Geometry: final body of the model. Coordinates: model frame, mm. Give positions to 0.01 mm unless a question says otherwise; leave off trailing zeros. Write each loop counter-clockwise with the first axis right and the second up, starting at its lowest first coordinate (ties: lowest second). Pieces come first, ordered by that corner, then holes. Notation, with made-up numbers: (24, 27) -> (50, 27) arc R29 ccw to (50, 54) -> close; hole circle Ø10 at (-1, 36). An arc over 180 degrees is marked (long way). Answer as a JSON object with one key per item and string values. Group by question number.
(1) Material intervals for probe 1 along X at (y, z) = (0.3, -2.5); probe 2 along Z at (x, y) = (2, 0.45); probe 3 along Y at (x, z) = (7.75, -205.5), sorted ascending.
(2) Contact query for a flat-ended pin moving along its axis: pin 1 Ø1.4 at (x, z) = (2, -2.5) entering from -Y. Output: stop coordinate, or through.
(3) Section query A-A on z = -196. Output: boundary loops of the cut face in (x, y).
Autodesk Inventor part; units mm, degrees
ref_plane "YZ Plane" through (0, 0, 0) normal (1, 0, 0) x (0, 1, 0)
ref_plane "XZ Plane" through (0, 0, 0) normal (0, 1, 0) x (-1, 0, 0)
ref_plane "XY Plane" through (0, 0, 0) normal (0, 0, 1) x (1, 0, 0)
sketch "草图1" plane through (0, 0, 0) normal (0, 1, 0) x (-1, 0, 0)
  line L0 (0, 0) -> (-10, 0)
  line L1 (-10, 0) -> (-10, -400)
  line L2 (-10, -400) -> (0, -400)
  line L3 (0, -400) -> (0, 0)
  dimension "d0" = 10
  dimension "d1" = 400
extrude "拉伸1" add sketch "草图1" along normal blind 1
sketch "草图2" plane through (0, 1, 0) normal (0, 1, 0) x (1, 0, 0)
  circle A0 centre (2, 2.5) radius 1.5
  circle A1 centre (8, 2.5) radius 1.5
  line L0 (0, 400) -> (0, 0)
  line L1 (10, 0) -> (10, 400)
  line L2 (0, 0) -> (10, 0)
  dimension "d4" = 3
  dimension "d5" = 3
  dimension "d6" = 2
  dimension "d7" = 2
  dimension "d8" = 2.5
  dimension "d9" = 2.5
sketch "草图3" plane through (0, 1, 0) normal (0, 1, 0) x (1, 0, 0)
  point P0 (0, 0)
extrude "拉伸2" add sketch "草图2" along normal blind 0.1
sketch "草图4" plane through (2, 1.1, -2.5) normal (0, 1, 0) x (1, 0, 0)
  circle A0 centre (0, 0) radius 1.5
  circle A1 centre (0, 0) radius 0.75
  circle A2 centre (6, 0) radius 1.5
  circle A3 centre (6, 0) radius 0.75
  point P0 (-2, -2.5)
  dimension "d12" = 1.5
  dimension "d13" = 1.5
extrude "拉伸3" cut sketch "草图4" against normal blind 3.85 contours A1 | A3
sketch "草图5" plane through (0, 1, 0) normal (0, 1, 0) x (1, 0, 0)
  line L0 (3.0005, 45) -> (4.4505, 45)
  line L1 (4.4505, 45) -> (4.4505, 395)
  line L2 (4.4505, 395) -> (3.0005, 395)
  line L3 (3.0005, 395) -> (3.0005, 45)
  line L4 (5.5405, 45) -> (6.9905, 45)
  line L5 (6.9905, 45) -> (6.9905, 395)
  line L6 (6.9905, 395) -> (5.5405, 395)
  line L7 (5.5405, 395) -> (5.5405, 45)
  line L8 (0, 0) -> (10, 0)
  line L9 (10, 400) -> (0, 400)
  line L10 (0, 400) -> (0, 0)
  dimension "d16" = 1.45
  dimension "d17" = 350
  dimension "d18" = 1.45
  dimension "d19" = 350
  dimension "d20" = 45
  dimension "d21" = 5
  dimension "d22" = 1.09
  dimension "d23" = 3.0005
extrude "拉伸4" add sketch "草图5" along normal blind 0.1
equation "\"折弯半径\" = 厚度"
equation "\"折弯释压宽度\" = 厚度"
equation "\"折弯释压深度\" = 0.5 * 厚度"
equation "\"拐角释压尺寸\" = 4 * 厚度"
equation "\"最小余量\" = 2 * 厚度"
equation "\"过渡半径\" = 折弯半径"
equation "\"Jacobi半径尺寸\" = 折弯半径"
equation "\"间隙大小\" = 厚度"
properties part number "Dosyn Rail"
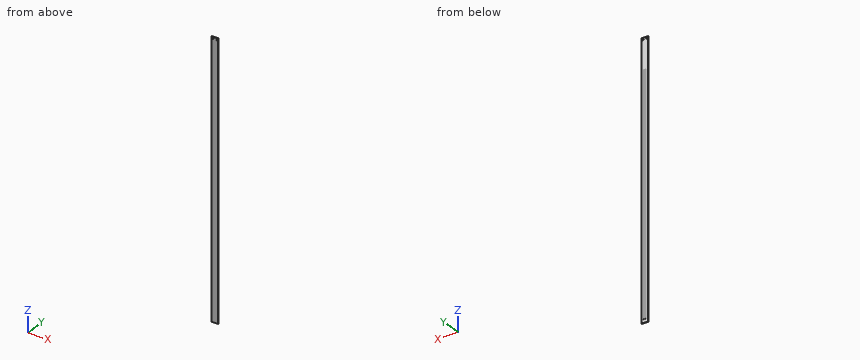
Answer list:
{
 "1": {"probe 1": "0 to 1.25, 2.75 to 7.25, 8.75 to 10", "probe 2": "-400 to -3.25, -1.75 to 0", "probe 3": "0 to 1"},
 "2": {"pin 1": "through"},
 "3": {"outline": "(0, 0) -> (10, 0) -> (10, 1) -> (6.99, 1) -> (6.99, 1.1) -> (5.54, 1.1) -> (5.54, 1) -> (4.45, 1) -> (4.45, 1.1) -> (3, 1.1) -> (3, 1) -> (0, 1) -> close"}
}
